Geometry: final body of the model. Coordinates: model frame, mm. Face numbers are marked on the shaded views. A direction names the side the tool comes from. Give positions to 0.01 mm unless a question says otherwise; leave off trailing zeros. Write each loop counter-clockwise with the first axis right and the second up, starting at its lowest first coordinate (ties: lowest second). Pieces come first, ordered by that corner, then holes. Notation, with made-up numbers: (15.5, 40.5) -> (24.5, 40.5) arc R16 ccw to (24.5, 63.5) -> close; hole circle Ø7 at (59.25, 76). An arc over 180 degrees is marked (long way). Answer in a Markdown table with one row per item. Add a question column.
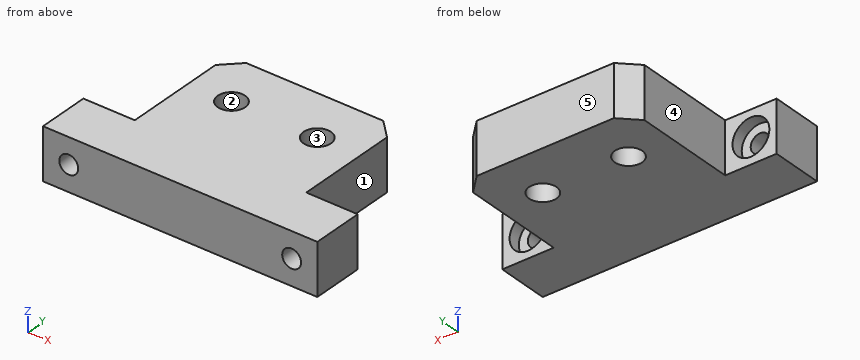
from build123d import *

# Parameters (mm, degrees)
SKETCH2_R                        = 8
CORPO_FUROS_20MM_DEPTH           = 30
CHANFROS_10X45_SIZE              = 10
REBAIXO_PARAFUSO_M10_D           = 11
REBAIXO_PARAFUSO_M10_CBORE_D     = 21.48
REBAIXO_PARAFUSO_M10_CBORE_DEPTH = 6.85


with BuildPart() as part:
    # Sketch2 → Corpo - Furos 20mm (new body)
    with BuildSketch(Plane.XY):
        Polygon((80, 0), (-80, 0), (-80, 30), (-50, 30), (-50, 100), (0, 100), (50, 100), (50, 30), (80, 30), align=None)
        with Locations((-25, 70)):
            Circle(SKETCH2_R, mode=Mode.SUBTRACT)
        with Locations(Location((25, 70, 0), (0, 0, 180))):
            Circle(SKETCH2_R, mode=Mode.SUBTRACT)
    extrude(amount=CORPO_FUROS_20MM_DEPTH)

    # Chanfros 10x45°
    chanfros_10x45_edges = [part.edges().sort_by_distance(p)[0] for p in [
        (50, 100, 15),
        (-50, 100, 15),
    ]]
    chamfer(chanfros_10x45_edges, length=CHANFROS_10X45_SIZE)

    # Rebaixo Parafuso M10 (through all)
    with Locations(Plane(origin=(0, 30, 0), x_dir=(1, 0, 0), z_dir=(0, 1, 0))):
        with Locations((-65, -15), (65, -15)):
            CounterBoreHole(REBAIXO_PARAFUSO_M10_D / 2, REBAIXO_PARAFUSO_M10_CBORE_D / 2, REBAIXO_PARAFUSO_M10_CBORE_DEPTH)


solid = part.part
Q1. Section C-C on z = 15. Return loops of the section in (x, y).
Q2. Section A-A on y = 70. Return loops of the section in (x, z), and give its area (3 significant figures).
Q3. Line query: probe 1 along X at (y, z) = (70.5, 22.75); probe 2 along Z at (x, y) = (65, 28.75); probe 3 along X at (y, z) = (10, 11.75). Output: solid intervals per line, ascending. Write a range as from..to.
Q4. Section D-D on z = 27.75. Return loops of the section in (x, y), and give its area (3 significant figures).
Q5. Contact query for flat-ended pins moving along their axis: pin 1 Ø6.5 at (x, z) = (-61, 11) entering from +Y; pin 2 Ø5 at (y, z) = (39.5, 9) entering from -X; pin 3 Ø14.5 at (x, y) = (-25, 70) entering from +Z; pin 4 Ø9 at (y, z) = (50.5, 22) entering from +X. Output: stop coordinate, or through.
Q6. Section B-B on x = 25. Return loops of the section in (y, z).
Q7. Access query for the marked faces 1 and 2. Directions: +Z, -Z, +X, -X, +Y, -Y. A direction counts if a zero-diameter tool reaches every point of the face in a straight line with its end or side. Return the directions, or none.
Q8. Pull-direction query (X, two-part tool) for the marked faces 3, 4 and 5; classes: +X half, -X half, draft (parallel to the pull), parting line (faces both ways), or undercut.
Checks:
| question | item | result |
|---|---|---|
| 1 | outline | (-80, 0) -> (-70.5, 0) -> (-70.5, 23.15) -> (-75.74, 23.15) -> (-75.74, 30) -> (-80, 30) -> close; (-59.5, 0) -> (59.5, 0) -> (59.5, 23.15) -> (54.26, 23.15) -> (54.26, 30) -> (50, 30) -> (50, 90) -> (40, 100) -> (-40, 100) -> (-50, 90) -> (-50, 30) -> (-54.26, 30) -> (-54.26, 23.15) -> (-59.5, 23.15) -> close; (70.5, 0) -> (80, 0) -> (80, 30) -> (75.74, 30) -> (75.74, 23.15) -> (70.5, 23.15) -> close; hole circle Ø16 at (-25, 70); hole circle Ø16 at (25, 70) |
| 2 | outline | (-50, 0) -> (-33, 0) -> (-33, 30) -> (-50, 30) -> close; (-17, 0) -> (17, 0) -> (17, 30) -> (-17, 30) -> close; (33, 0) -> (50, 0) -> (50, 30) -> (33, 30) -> close |
| 2 | area | 2,040 mm^2 |
| 3 | probe 1 | -50..-32.98, -17.02..17.02, 32.98..50 |
| 3 | probe 2 | 0..4.26, 25.74..30 |
| 3 | probe 3 | -80..-69.44, -60.56..60.56, 69.44..80 |
| 4 | outline | (-80, 0) -> (80, 0) -> (80, 30) -> (50, 30) -> (50, 90) -> (40, 100) -> (-40, 100) -> (-50, 90) -> (-50, 30) -> (-80, 30) -> close; hole circle Ø16 at (-25, 70); hole circle Ø16 at (25, 70) |
| 4 | area | 11,300 mm^2 |
| 5 | pin 1 | y = 23.15 |
| 5 | pin 2 | x = -50 |
| 5 | pin 3 | through |
| 5 | pin 4 | x = 50 |
| 6 | outline | (0, 0) -> (62, 0) -> (62, 30) -> (0, 30) -> close; (78, 0) -> (100, 0) -> (100, 30) -> (78, 30) -> close |
| 7 | face 1 | +Z, -Z, +X, +Y |
| 7 | face 2 | +Z, -Z |
| 8 | face 3 | undercut |
| 8 | face 4 | -X half |
| 8 | face 5 | draft |
